Design review of the part built by this model. Coordinates are the model's own, in mm. Coordinates: 2 decimals unless noted, no trailing zeros. Answer as a JSON object with one key per item and string values.
Autodesk Inventor part; units mm, degrees
ref_plane "side_4d_XY" through (-20, 0, -310) normal (-1, 0, 0) x (0, 1, 0)
ref_plane "side_4d_YZ" through (-20, 0, -310) normal (0, 1, 0) x (0, 0, -1)
ref_plane "side_4d_ZX" through (-20, 0, -310) normal (0, 0, -1) x (-1, 0, 0)
sketch "Skizze_1" plane through (0, 0, 0) normal (0, 0, 1) x (1, 0, 0)
  arc A0 (-20, -17) -> (-17, -20) centre (-17, -17) ccw
  line L0 (-17, -20) -> (-4.1, -20)
  line L1 (-4.1, -20) -> (-4.1, -17)
  line L2 (-4.1, -17) -> (-10.5, -17)
  line L3 (-10.5, -17) -> (-10.5, -13.6627)
  arc A1 (-10.0314, -12.5314) -> (-10.5, -13.6627) centre (-8.9002, -13.6627) ccw
  line L4 (-10.0314, -12.5314) -> (-7.4645, -9.9645)
  arc A2 (-3.9289, -8.5) -> (-7.4645, -9.9645) centre (-3.9289, -13.5) ccw
  line L5 (-3.9289, -8.5) -> (3.9289, -8.5)
  arc A3 (7.4645, -9.9645) -> (3.9289, -8.5) centre (3.9289, -13.5) ccw
  line L6 (7.4645, -9.9645) -> (10.0314, -12.5314)
  arc A4 (10.5, -13.6627) -> (10.0314, -12.5314) centre (8.9002, -13.6627) ccw
  line L7 (10.5, -13.6627) -> (10.5, -17)
  line L8 (10.5, -17) -> (4.1, -17)
  line L9 (4.1, -17) -> (4.1, -20)
  line L10 (4.1, -20) -> (17, -20)
  arc A5 (17, -20) -> (20, -17) centre (17, -17) ccw
  line L11 (20, -17) -> (20, -4.1)
  line L12 (20, -4.1) -> (17, -4.1)
  line L13 (17, -4.1) -> (17, -10.5)
  line L14 (17, -10.5) -> (13.6627, -10.5)
  arc A6 (12.5314, -10.0314) -> (13.6627, -10.5) centre (13.6627, -8.9002) ccw
  line L15 (12.5314, -10.0314) -> (9.9645, -7.4645)
  arc A7 (8.5, -3.9289) -> (9.9645, -7.4645) centre (13.5, -3.9289) ccw
  line L16 (8.5, -3.9289) -> (8.5, 3.9289)
  arc A8 (9.9645, 7.4645) -> (8.5, 3.9289) centre (13.5, 3.9289) ccw
  line L17 (9.9645, 7.4645) -> (12.5314, 10.0314)
  arc A9 (13.6627, 10.5) -> (12.5314, 10.0314) centre (13.6627, 8.9002) ccw
  line L18 (13.6627, 10.5) -> (17, 10.5)
  line L19 (17, 10.5) -> (17, 4.1)
  line L20 (17, 4.1) -> (20, 4.1)
  line L21 (20, 4.1) -> (20, 17)
  arc A10 (20, 17) -> (17, 20) centre (17, 17) ccw
  line L22 (17, 20) -> (4.1, 20)
  line L23 (4.1, 20) -> (4.1, 17)
  line L24 (4.1, 17) -> (10.5, 17)
  line L25 (10.5, 17) -> (10.5, 13.6627)
  arc A11 (10.0314, 12.5314) -> (10.5, 13.6627) centre (8.9002, 13.6627) ccw
  line L26 (10.0314, 12.5314) -> (7.4645, 9.9645)
  arc A12 (3.9289, 8.5) -> (7.4645, 9.9645) centre (3.9289, 13.5) ccw
  line L27 (3.9289, 8.5) -> (-3.9289, 8.5)
  arc A13 (-7.4645, 9.9645) -> (-3.9289, 8.5) centre (-3.9289, 13.5) ccw
  line L28 (-7.4645, 9.9645) -> (-10.0314, 12.5314)
  arc A14 (-10.5, 13.6627) -> (-10.0314, 12.5314) centre (-8.9002, 13.6627) ccw
  line L29 (-10.5, 13.6627) -> (-10.5, 17)
  line L30 (-10.5, 17) -> (-4.1, 17)
  line L31 (-4.1, 17) -> (-4.1, 20)
  line L32 (-4.1, 20) -> (-17, 20)
  arc A15 (-17, 20) -> (-20, 17) centre (-17, 17) ccw
  line L33 (-20, 17) -> (-20, 4.1)
  line L34 (-20, 4.1) -> (-17, 4.1)
  line L35 (-17, 4.1) -> (-17, 10.5)
  line L36 (-17, 10.5) -> (-13.6627, 10.5)
  arc A16 (-12.5314, 10.0314) -> (-13.6627, 10.5) centre (-13.6627, 8.9002) ccw
  line L37 (-12.5314, 10.0314) -> (-9.9645, 7.4645)
  arc A17 (-8.5, 3.9289) -> (-9.9645, 7.4645) centre (-13.5, 3.9289) ccw
  line L38 (-8.5, 3.9289) -> (-8.5, -3.9289)
  arc A18 (-9.9645, -7.4645) -> (-8.5, -3.9289) centre (-13.5, -3.9289) ccw
  line L39 (-9.9645, -7.4645) -> (-12.5314, -10.0314)
  arc A19 (-13.6627, -10.5) -> (-12.5314, -10.0314) centre (-13.6627, -8.9002) ccw
  line L40 (-13.6627, -10.5) -> (-17, -10.5)
  line L41 (-17, -10.5) -> (-17, -4.1)
  line L42 (-17, -4.1) -> (-20, -4.1)
  line L43 (-20, -4.1) -> (-20, -17)
  circle A20 centre (0, 0) radius 6
extrude "Extrusion1" add sketch "Skizze_1" against normal blind 620
sketch "Sketch2" plane through (0, 0, 0) normal (0, 0, 1) x (1, 0, 0)
  point P0 (-15, -15)
hole "Drilling 1" at (-15, -15, 0) direction (0, 0, -1) diameter 5 depth 6000
sketch "Sketch3" plane through (0, 0, 0) normal (0, 0, 1) x (1, 0, 0)
  point P0 (15, -15)
hole "Drilling 2" at (15, -15, 0) direction (0, 0, -1) diameter 5 depth 6000
sketch "Sketch4" plane through (0, 0, 0) normal (0, 0, 1) x (1, 0, 0)
  point P0 (15, 15)
hole "Drilling 3" at (15, 15, 0) direction (0, 0, -1) diameter 5 depth 6000
sketch "Sketch5" plane through (0, 0, 0) normal (0, 0, 1) x (1, 0, 0)
  point P0 (-15, 15)
hole "Drilling 4" at (-15, 15, 0) direction (0, 0, -1) diameter 5 depth 6000
ref_plane "side_4d_XY" through (-20, 0, -310) normal (-1, 0, 0) x (0, 1, 0)
ref_plane "side_4d_YZ" through (-20, 0, -310) normal (0, 1, 0) x (0, 0, -1)
ref_plane "side_4d_ZX" through (-20, 0, -310) normal (0, 0, -1) x (-1, 0, 0)
ref_plane "side_1a_XY" through (0, 20, -310) normal (0, 1, 0) x (1, 0, 0)
ref_plane "side_1a_YZ" through (0, 20, -310) normal (1, 0, 0) x (0, 0, -1)
ref_plane "side_1a_ZX" through (0, 20, -310) normal (0, 0, -1) x (0, 1, 0)
ref_plane "side_2b_XY" through (20, 0, -310) normal (1, 0, 0) x (0, -1, 0)
ref_plane "side_2b_YZ" through (20, 0, -310) normal (0, -1, 0) x (0, 0, -1)
ref_plane "side_2b_ZX" through (20, 0, -310) normal (0, 0, -1) x (1, 0, 0)
ref_plane "side_3c_XY" through (0, -20, -310) normal (0, -1, 0) x (-1, 0, 0)
ref_plane "side_3c_YZ" through (0, -20, -310) normal (-1, 0, 0) x (0, 0, -1)
ref_plane "side_3c_ZX" through (0, -20, -310) normal (0, 0, -1) x (0, -1, 0)
ref_plane "end_XY" through (0, 0, -620) normal (0, 0, -1) x (1, 0, 0)
ref_plane "end_YZ" through (0, 0, -620) normal (1, 0, 0) x (0, -1, 0)
ref_plane "end_ZX" through (0, 0, -620) normal (0, -1, 0) x (0, 0, -1)
ref_plane "start_XY" through (0, 0, 0) normal (0, 0, 1) x (1, 0, 0)
ref_plane "start_YZ" through (0, 0, 0) normal (1, 0, 0) x (0, 1, 0)
ref_plane "start_ZX" through (0, 0, 0) normal (0, 1, 0) x (0, 0, 1)
properties part number "MayTec 1.11.040040.43S_Profile 40x40, 4E, S_620_Detail_(0;0,0,0)"
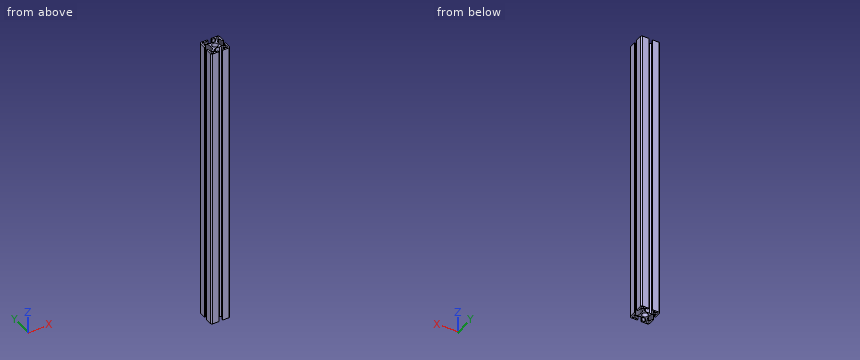
1) Clearance check with flat-ended pins moving along their axes: pin 1 Ø1.5 at (x, z) = (0, -159) entering from +Y; pin 2 Ø2 at (y, z) = (1, -84.5) entering from -X; pin 3 Ø2.5 at (y, z) = (-18.5, -329.5) entering from -X. State where each tip first meets the part, or that it passes through.
Completed:
{"pin 1": "y = 8.5", "pin 2": "x = -8.5", "pin 3": "x = -19.99"}
2) Add section A-A, the plane z = -121.5. Count the separate pieces of the cut face and the enclosed holes in it, and give its area (3 significant figures).
Completed:
{"separate pieces": "1", "enclosed holes": "5", "area": "674 mm²"}
3) Wall thickness on probe 1 along Y at (x, z) = (15, -138); probe 2 along Y at (x, z) = (7.5, -317.5): over which ranges is each line inside the solid? List them lowest first.
Completed:
{"probe 1": "-20 to -17.5, -12.5 to -10.5, 10.5 to 12.5, 17.5 to 20", "probe 2": "-20 to -17, -10 to 10, 17 to 20"}
